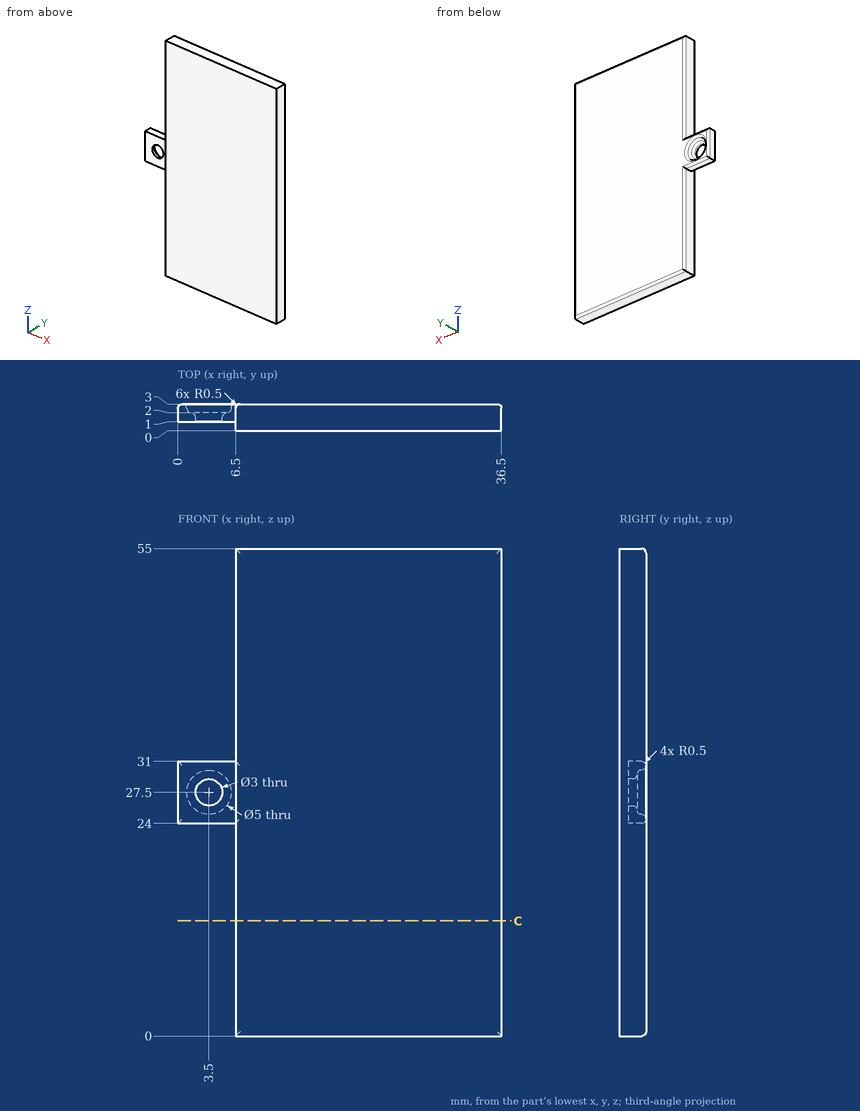
Verification items for this drawing (mm, ordinates from the low corner). Give positions to 0.01 mm unless a question says otherwise; leave off trailing zeros. Write each loop counter-clockwise with the first axis right and the second up, starting at its lowest first coordinate (ties: lowest second). Pieces come first, ordered by that corner, then holes.
1) Cross-section at C-C (z = 13). Record the boundary of the cut face in (x, y), plus the area to 3 significant figures.
Values follow:
outline: (6.5, 0) - (36.5, 0) - (36.5, 2.5) arc R0.5 ccw to (36, 3) - (7, 3) arc R0.5 ccw to (6.5, 2.5) - close
area: 89.9 mm2
2) Thickness scan on line 1 (X direction, y = 1.35, z = 27.5); line 2 (X direction, y = 2.55, z = 27.5); line 3 (X direction, y = 1.65, z = 43). Record the ranges inside material, lowest first.
Values follow:
line 1: x = 0 to 2, 5 to 36.5
line 2: x = 0 to 1, 6 to 36.5
line 3: x = 6.5 to 36.5
3) Go/stop test with flat-tipped pins: pin 1 Ø4 at (x, z) = (3.5, 27.5) entering from -Y; pin 2 Ø1.2 at (x, y) = (4.5, 2) entering from -Z; pin 3 Ø4.5 at (x, z) = (4, 27.5) entering from +Y; pin 4 Ø1.5 at (x, z) = (22.5, 36.5) entering from -Y. Record where each tip stops, or that it passes through.
Values follow:
pin 1: stops at y = 1
pin 2: stops at z = 24
pin 3: stops at y = 2.93
pin 4: stops at y = 0
